from build123d import *

# Parameters (mm, degrees)
BOSS_EXTRUDE1_DEPTH      = 137.5
BOSS_EXTRUDE1_DEPTH_BACK = 137.5
SKETCH2_R                = 2
CUT_EXTRUDE1_DEPTH       = 139.225359468
CHAMFER1_SIZE            = 1


with BuildPart() as part:
    # Sketch1 → Boss-Extrude1 (new, two sides: drawn at the far end of the back side and taken through both)
    with BuildSketch(Plane(origin=(0, 0, 0), x_dir=(0, 0, -1), z_dir=(1, 0, 0)).offset(-BOSS_EXTRUDE1_DEPTH_BACK)):
        with BuildLine():
            Line((0, -10), (0, -0.5))
            ThreePointArc((0, -0.5), (0.146446609, -0.146446609), (0.5, 0))
            Line((0.5, 0), (10, 0))
            Line((10, 0), (10, -2))
            Line((10, -2), (2.5, -2))
            ThreePointArc((2.5, -2), (2.146446609, -2.146446609), (2, -2.5))
            Line((2, -2.5), (2, -10))
            Line((2, -10), (0, -10))
        make_face()
    extrude(amount=BOSS_EXTRUDE1_DEPTH + BOSS_EXTRUDE1_DEPTH_BACK)

    # Sketch2 → Cut-Extrude1 (cut, through all)
    with BuildSketch(Plane.XY):
        with Locations((-120, -6)):
            Circle(SKETCH2_R)
        with Locations((-40, -6)):
            Circle(SKETCH2_R)
        with Locations((40, -6)):
            Circle(SKETCH2_R)
        with Locations((120, -6)):
            Circle(SKETCH2_R)
    extrude(amount=-CUT_EXTRUDE1_DEPTH, mode=Mode.SUBTRACT)

    # Chamfer1
    chamfer1_edges = [part.edges().sort_by_distance(p)[0] for p in [
        (-122, -6, -2),
        (-42, -6, -2),
        (38, -6, -2),
        (118, -6, -2),
    ]]
    chamfer(chamfer1_edges, length=CHAMFER1_SIZE)


solid = part.part
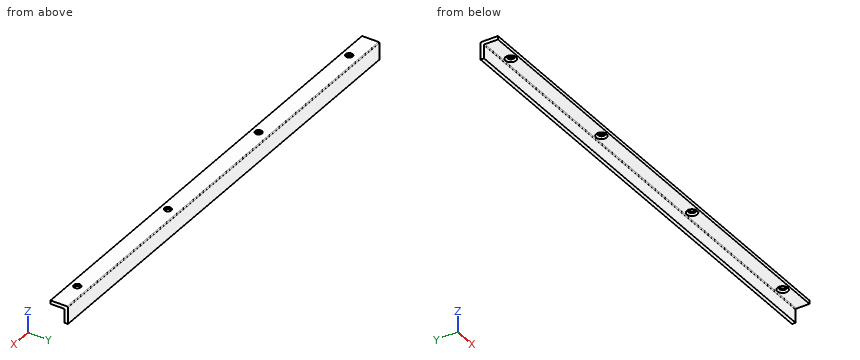
The listing builds one solid part. Answer for the finished solid, in the listing's coordinates (mm). Give positions to 0.01 mm unless a question says otherwise; leave off trailing zeros. Order: outer loops, then holes, each group sorted by start corner. A loop starts at its lowest first (then second) coordinate and runs counter-clockwise, first axis right, second up. Notation, with made-up numbers: (-32, -37.5) - (-7, -37.5) arc R18 ccw to (-7, -31.5) - close; hole circle Ø6 at (66.5, 82.25). An arc over 180 degrees is marked (long way). One line per item, written item: value. Start each with the question number.
1) Find the intervals of material crossed by L1, parallel to X at y = -4.5, z = -1.5; L2, parallel to Y at x = 40, z = -0.65; L3, parallel to Y at x = 35, z = -8.5, in increasing order.
2) Given pin 1 Ø1.5 at (x, z) = (-12, -2.5) entering from -Y; pin 2 Ø2 at (x, z) = (-57, -5) entering from -Y; pin 3 Ø2 at (x, y) = (85, -7.5) entering from -Z, each flat-ended and moving along its own axis, determine where each tip first touches the part or whether it passes through.
3) A cutting plane is placed at A-A on y = -6. Give the vertices of the cut face in (x, z), then the cut area to 3 significant figures.
4) A cutting plane is placed at C-C on z = -5.75. Give the vertices of the cut face in (x, y), then the cut area to 3 significant figures.
5) A cutting plane is placed at B-B on x = 112. Give the vertices of the cut face in (y, z), then the cut area to 3 significant figures.
Answer sheet:
1. L1: x = -137.5 to -122, -118 to -42, -38 to 38, 42 to 118, 122 to 137.5
1. L2: y = -10 to -8, -4 to 0
1. L3: y = -2 to 0
2. pin 1: stops at y = -10
2. pin 2: stops at y = -2
2. pin 3: stops at z = -2
3. outline: (-137.5, -2) - (-123, -2) - (-122, -1) - (-122, 0) - (-137.5, 0) - close; (-118, -1) - (-117, -2) - (-43, -2) - (-42, -1) - (-42, 0) - (-118, 0) - close; (-38, -1) - (-37, -2) - (37, -2) - (38, -1) - (38, 0) - (-38, 0) - close; (42, -1) - (43, -2) - (117, -2) - (118, -1) - (118, 0) - (42, 0) - close; (122, -1) - (123, -2) - (137.5, -2) - (137.5, 0) - (122, 0) - close
3. area: 514 mm2
4. outline: (-137.5, -2) - (137.5, -2) - (137.5, 0) - (-137.5, 0) - close
4. area: 550 mm2
5. outline: (-10, -2) - (-2.5, -2) arc R0.5 cw to (-2, -2.5) - (-2, -10) - (0, -10) - (0, -0.5) arc R0.5 ccw to (-0.5, 0) - (-10, 0) - close
5. area: 36.0 mm2
